```python
from build123d import *

# Parameters (mm, degrees)
SKETCH1_R           = 31
BOSS_EXTRUDE1_DEPTH = 20
SKETCH2_R           = 31
SKETCH2_R_2         = 28
CUT_EXTRUDE1_DEPTH  = 16
SKETCH3_R           = 4
CUT_EXTRUDE2_DEPTH  = 21


with BuildPart() as part:
    # Sketch1 → Boss-Extrude1 (new body)
    with BuildSketch(Plane(origin=(0, 0, 0), x_dir=(0, 1, 0), z_dir=(0, 0, 1))):
        Circle(SKETCH1_R)
    extrude(amount=BOSS_EXTRUDE1_DEPTH)

    # Sketch2 → Cut-Extrude1 (cut)
    with BuildSketch(Plane(origin=(0, 0, 2), x_dir=(0, 1, 0), z_dir=(0, 0, 1))):
        Circle(SKETCH2_R)
        Circle(SKETCH2_R_2, mode=Mode.SUBTRACT)
    extrude(amount=CUT_EXTRUDE1_DEPTH, mode=Mode.SUBTRACT)

    # Sketch3 → Cut-Extrude2 (cut, through all)
    with BuildSketch(Plane.XY.offset(20)):
        Circle(SKETCH3_R)
    extrude(amount=-CUT_EXTRUDE2_DEPTH, mode=Mode.SUBTRACT)


solid = part.part
```
CAD build for the part. Positions are in the model's coordinates, mm. A direction names the side the tool comes from. Coordinates: 2 decimals unless noted, no trailing zeros. Order: outer loops, then holes, each group sorted by start corner. A loop starts at its lowest first (then second) coordinate and runs counter-clockwise, first axis right, second up.
(1) Saw through at C-C, the plane z = 8.5. Write the cut outline in (x, y), and give its area (3 significant figures).
Solution:
outline: circle Ø56 at (0, 0); hole circle Ø8 at (0, 0)
area: 2,410 mm2
(2) Pin check, flat tips, straight feed: pin 1 Ø6 at (y, z) = (-20.5, 9) entering from +X; pin 2 Ø10 at (y, z) = (21, 7.5) entering from -X; pin 3 Ø6.5 at (x, y) = (0, 0) entering from -Z; pin 4 Ø5 at (y, z) = (3, 11) entering from +X. Stop position of each tip, or through.
Solution:
pin 1: stops at x = 21.86
pin 2: stops at x = -22.98
pin 3: passes through
pin 4: stops at x = 28
(3) Saw through at A-A, the plane y = 0. Write the cut outline in (x, z).
Solution:
outline: (-31, 0) - (-4, 0) - (-4, 20) - (-31, 20) - (-31, 18) - (-28, 18) - (-28, 2) - (-31, 2) - close; (4, 0) - (31, 0) - (31, 2) - (28, 2) - (28, 18) - (31, 18) - (31, 20) - (4, 20) - close
(4) Drill centre lines: L1, parallel to Z at x = 22.5, y = 18.5; L2, parallel to Y at x = 0, z = 13.25; L3, parallel to X at y = -1, z = 12.5. Where is each one in solid material? Low to high.
Solution:
L1: z = 0 to 2, 18 to 20
L2: y = -28 to -4, 4 to 28
L3: x = -27.98 to -3.87, 3.87 to 27.98
(5) Which spindle directions (+Z, -Z, +X, -X, +Y, -Y) get a long thin tool onto all of the face, cutting with end or side? Do faces 4 (the face through (27.4, -7, 2)), 5 (the face through (6, 0, 0)). Say none if no direction does.
Solution:
face 4: none
face 5: -Z, +X, -X, +Y, -Y
(6) Mould opens along Y. For faces 1 (the face through (-0.867, -3.905, 10.14)), 2 (the face through (27.4, -7, 18)), 3 (the face through (-30.736, -4.036, 18.986)) say: released by +Y, released by -Y, zero draft, split by the parting line, or undercut.
Solution:
face 1: undercut
face 2: zero draft
face 3: split by the parting line
(7) Saw through at D-D, the plane y = -17.5. Write the cut outline in (x, z), and give its area (3 significant figures).
Solution:
outline: (-25.59, 0) - (25.59, 0) - (25.59, 2) - (21.86, 2) - (21.86, 18) - (25.59, 18) - (25.59, 20) - (-25.59, 20) - (-25.59, 18) - (-21.86, 18) - (-21.86, 2) - (-25.59, 2) - close
area: 904 mm2
